```python
from build123d import *

# Parameters (mm, degrees)
F0_R     = 30
F1_DEPTH = 30
F2_R     = 4.9
F3_DEPTH = 30
F4_R     = 5.45
F5_DEPTH = 25


with BuildPart() as f1:
    # F0 (on Top) → F1 (new body)
    with BuildSketch(Plane.XY):
        Circle(F0_R)
    extrude(amount=F1_DEPTH)

    # F2 (on face) → F3 (cut, through all)
    with BuildSketch(Plane.XY.offset(30)):
        Circle(F2_R)
        with Locations((0, 18)):
            Circle(F2_R)
        with Locations((-15.588457, 9)):
            Circle(F2_R)
        with Locations((-15.588457, -9)):
            Circle(F2_R)
        with Locations((0, -18)):
            Circle(F2_R)
        with Locations((15.588457, -9)):
            Circle(F2_R)
        with Locations((15.588457, 9)):
            Circle(F2_R)
    extrude(amount=-F3_DEPTH, mode=Mode.SUBTRACT)

    # F4 (on face) → F5 (cut)
    with BuildSketch(Plane.XY.offset(30)):
        Circle(F4_R)
        with Locations((0, 18)):
            Circle(F4_R)
        with Locations((-15.588457, 9)):
            Circle(F4_R)
        with Locations((-15.588457, -9)):
            Circle(F4_R)
        with Locations((0, -18)):
            Circle(F4_R)
        with Locations((15.588457, -9)):
            Circle(F4_R)
        with Locations((15.588457, 9)):
            Circle(F4_R)
    extrude(amount=-F5_DEPTH, mode=Mode.SUBTRACT)


solid = f1.part
```
Geometry: final body of the model. Coordinates: model frame, mm. A direction names the side the tool comes from. Round coordinates to 2 decimals unless told otherwise and drop trailing zeros. Write each loop counter-clockwise with the first axis right and the second up, starting at its lowest first coordinate (ties: lowest second). Pieces come first, ordered by that corner, then holes. Notation, with made-up numbers: M 80,25.5 L 93,25.5 A21 cw 93,60.5 Z; hole C -15.75,-4.5 d8. An arc over 180 degrees is marked long. Answer in a Markdown table with one row per item. Add a question column.
(1) Contact query for flat-ended pins moving along their axis: pin 1 (6 mm diameter, centred on x = -17.5, y = 24, fed in from -Z); pin 2 (2 mm diameter, centred on x = 20, z = 13.5, fed in from +Y); pin 3 (10 mm diameter, centred on y = 13.5, z = 6.5, fed in from -X); pin 4 (1.5 mm diameter, centred on y = -6, z = 20.5, fed in from -X). Output: stop coordinate, or through.
(2) Ray query, L1, parallel to Y at x = 0, z = 3.3; L2, parallel to Y at x = -16.5, z = 16.75; L3, parallel to Y at x = -16, z = 10.25. Return the intervals inside material, ascending.
(3) Cut plane B-B, the plane y = -18. Return the cut outline in (x, z).
(4) Cut plane D-D, the plane x = 16.5. Return the cut outline in (y, z).
(5) Reachability of faces 1 (the face through (-16.77, -14.32, 17.68)), 2 (the face through (-1.062, -22.783, 2.535)) from +Z, -Z, +X, -X, +Y, -Y: full face, straight path, thin tool, end or side. Return the list, or none.
(6) Cut plane A-A, the plane x = 0. Return the cut outline in (y, z), then the cut area to 4 significant figures.
(7) Cut plane C-C, the plane z = 14.75. Return the cut outline in (x, y).
(8) Draft query along Y for faces 3 (the face through (14.41, -14.32, 17.68)), 4 (the face through (-29.97, 1.32, 14.79)), 5 (the face through (14.41, 3.68, 17.68)), 6 (the face through (6, 0, 30)). Return one class per face: pulls with the +Y half, pulls with the -Y half, needs draft (parallel to the pull), parting line crosses it, or undercut.
Established:
| question | item | result |
|---|---|---|
| 1 | pin 1 | z = 0 |
| 1 | pin 2 | y = 23.22 |
| 1 | pin 3 | x = -28.77 |
| 1 | pin 4 | x = -29.54 |
| 2 | L1 | -30 to -22.9, -13.1 to -4.9, 4.9 to 13.1, 22.9 to 30 |
| 2 | L2 | -25.05 to -14.37, -3.63 to 3.63, 14.37 to 25.05 |
| 2 | L3 | -25.38 to -14.43, -3.57 to 3.57, 14.43 to 25.38 |
| 3 | outline | M -24,0 L -4.9,0 L -4.9,5 L -5.45,5 L -5.45,30 L -24,30 Z; M 4.9,0 L 24,0 L 24,30 L 5.45,30 L 5.45,5 L 4.9,5 Z |
| 4 | outline | M -25.05,0 L -13.81,0 L -13.81,5 L -14.37,5 L -14.37,30 L -25.05,30 Z; M -4.19,0 L 4.19,0 L 4.19,5 L 3.63,5 L 3.63,30 L -3.63,30 L -3.63,5 L -4.19,5 Z; M 13.81,0 L 25.05,0 L 25.05,30 L 14.37,30 L 14.37,5 L 13.81,5 Z |
| 5 | face 1 | +Z |
| 5 | face 2 | +Z, -Z |
| 6 | outline | M -30,0 L -22.9,0 L -22.9,5 L -23.45,5 L -23.45,30 L -30,30 Z; M -13.1,0 L -4.9,0 L -4.9,5 L -5.45,5 L -5.45,30 L -12.55,30 L -12.55,5 L -13.1,5 Z; M 4.9,0 L 13.1,0 L 13.1,5 L 12.55,5 L 12.55,30 L 5.45,30 L 5.45,5 L 4.9,5 Z; M 22.9,0 L 30,0 L 30,30 L 23.45,30 L 23.45,5 L 22.9,5 Z |
| 6 | area | 835.5 mm² |
| 7 | outline | C 0,0 d60; hole C -15.59,-9 d10.9; hole C -15.59,9 d10.9; hole C 0,-18 d10.9; hole C 0,0 d10.9; hole C 0,18 d10.9; hole C 15.59,-9 d10.9; hole C 15.59,9 d10.9 |
| 8 | face 3 | undercut |
| 8 | face 4 | parting line crosses it |
| 8 | face 5 | undercut |
| 8 | face 6 | needs draft |
